Verification items for this drawing (mm, ordinates from the low corner). Round coordinates to 2 decimals unless told otherwise and drop trailing zeros. Loops run counter-clockwise (first coordinate to the right, second up) from the corner with the lowest first, then second, coordinate; pieces in that order, holes last. Notation, with made-up numbers: M 2.25,2 L 45.25,2 A20 cw 45.25,27 Z; hole C -15,1.25 d6. An arc over 180 degrees is marked long. Answer as CSV lines item,"result".
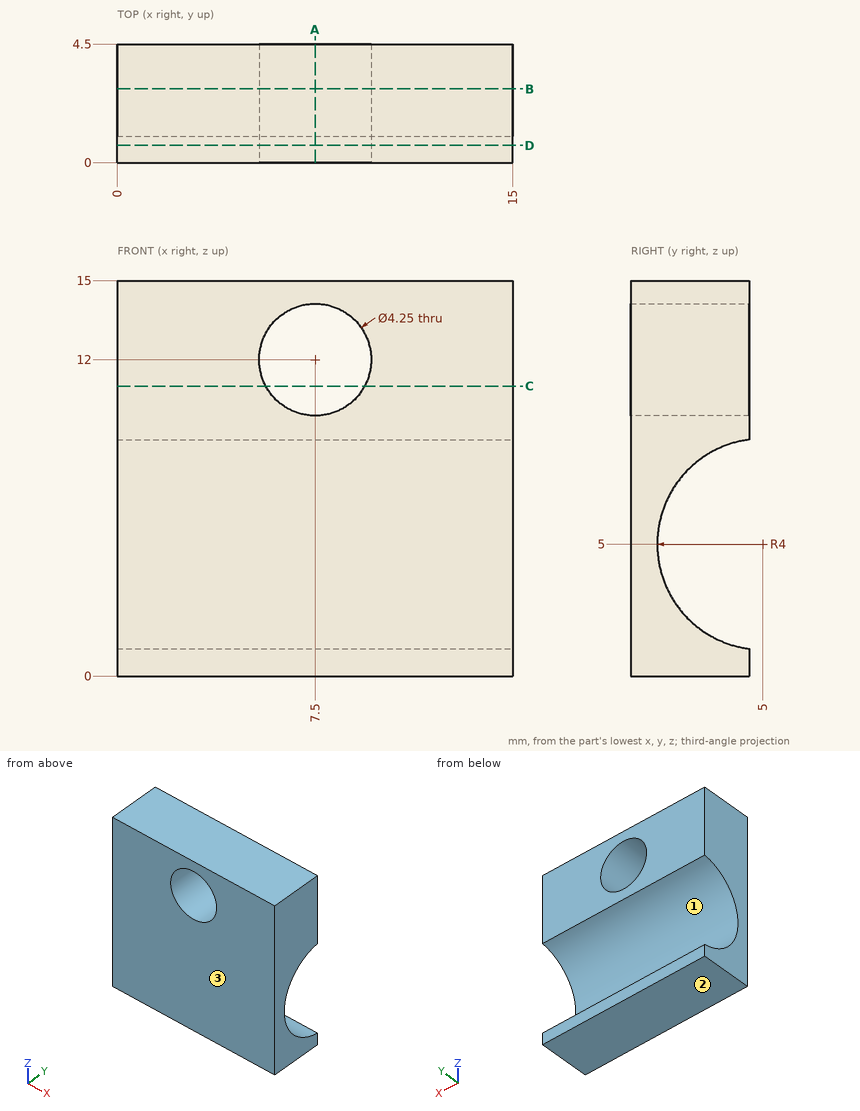
1) Section check B-B (y = 2.8). Record the cut outline in (x, z) (3 decimals).
Here are the results:
outline,"M 0,0 L 15,0 L 15,1.659 L 0,1.659 Z; M 0,8.341 L 15,8.341 L 15,15 L 0,15 Z; hole C 7.5,12 d4.25"
2) Draft check along Z on the marked faces 1, 2 and 3. Enter one of: +Z half, -Z half, draft (parallel to the pull), parting line (faces both ways), or undercut.
Here are the results:
face 1,"undercut"
face 2,"-Z half"
face 3,"draft"
3) Section check D-D (y = 0.65). Record the cut outline in (x, z) (3 decimals).
Here are the results:
outline,"M 0,0 L 15,0 L 15,15 L 0,15 Z; hole C 7.5,12 d4.25"
4) Material ranges on probe 1 along X at (y, z) = (2.65, 12) (3 decimals); probe 2 along Z at (x, y) = (7.25, 2.7); probe 3 along Y at (x, z) = (13.5, 4.5), recorded low to high.
Here are the results:
probe 1,"x = 0 to 5.375, 9.625 to 15"
probe 2,"z = 0 to 1.73, 8.27 to 9.89, 14.11 to 15"
probe 3,"y = 0 to 1.03"
5) Section check C-C (z = 11). Record the cut outline in (x, y) (3 decimals).
Here are the results:
outline,"M 0,0 L 5.625,0 L 5.625,4.5 L 0,4.5 Z; M 9.375,0 L 15,0 L 15,4.5 L 9.375,4.5 Z"
6) Section check A-A (x = 7.5). Record the cut outline in (y, z) (3 decimals).
Here are the results:
outline,"M 0,0 L 4.5,0 L 4.5,1.031 A4 cw 4.5,8.969 L 4.5,9.875 L 0,9.875 Z; M 0,14.125 L 4.5,14.125 L 4.5,15 L 0,15 Z"
